Autodesk Inventor part; units mm, degrees
ref_plane "YZ Plane" through (0, 0, 0) normal (1, 0, 0) x (0, 1, 0)
ref_plane "XZ Plane" through (0, 0, 0) normal (0, 1, 0) x (-1, 0, 0)
ref_plane "XY Plane" through (0, 0, 0) normal (0, 0, 1) x (1, 0, 0)
sketch "Sketch1" plane through (0, 0, 0) normal (0, 1, 0) x (-1, 0, 0)
  circle A0 centre (0, 0) radius 3
  line L0 (1.25, 1.75) -> (-1.25, 1.75)
  line L1 (-1.25, 1.75) -> (-1.25, -1.75)
  line L2 (-1.25, -1.75) -> (1.25, -1.75)
  line L3 (1.25, -1.75) -> (1.25, 1.75)
  dimension "d0" = 6
  dimension "d1" = 2.5
  dimension "d2" = 3.5
  dimension "d3" = 1.25
  dimension "d4" = 1.75
extrude "Extrusion1" add sketch "Sketch1" along normal blind 4 contours A0 | L3 L2 L1 L0
extrude "Extrusion2" cut sketch "Sketch1" along normal blind 3 contours L3 L2 L1 L0
fillet "Fillet1" radius 1 1 edges at (3, 4, 0)
properties part number "Power_Button"
For this review, take the finished solid that the model builds, in its own axes (mm). Round coordinates to 2 decimals unless told otherwise and drop trailing zeros. Loops run counter-clockwise (first coordinate to the right, second up) from the corner with the lowest first, then second, coordinate; pieces in that order, holes last. Notation, with made-up numbers: (-1, -0.75) - (15, -0.75) arc R22 cw to (15, 15.25) - close; hole circle Ø4 at (44.5, 32). An arc over 180 degrees is marked (long way). Use one line per item in the form item = value.
1) Mouldability with a two-part tool opening along X and no side actions: class faces 1 (the face through (1.25, 1, 0)), 2 (the face through (0, 4, 0)), 3 (the face through (3, 1, 0)) as pulls with the +X half, pulls with the -X half, needs draft (parallel to the pull), parting line crosses it, or undercut.
Solutions:
face_1 = undercut
face_2 = needs draft
face_3 = parting line crosses it
2) We need section C-C on x = 0. Write out the cut boundary in (y, z), then the cut area to 3 significant figures.
Solutions:
outline = (0, -3) - (3, -3) arc R1 ccw to (4, -2) - (4, 2) arc R1 ccw to (3, 3) - (0, 3) - (0, 1.75) - (3, 1.75) - (3, -1.75) - (0, -1.75) - close
area = 13.1 mm2
3) We need section A-A on y = 1.9. Write out the cut boundary in (x, z).
Solutions:
outline = circle Ø6 at (0, 0); hole (-1.25, -1.75) - (1.25, -1.75) - (1.25, 1.75) - (-1.25, 1.75) - close
4) We need section D-D on y = 3.3. Write out the cut boundary in (x, z), then the cut area to 3 significant figures.
Solutions:
outline = circle Ø5.91 at (0, 0)
area = 27.4 mm2
5) Wall thickness on probe 1 along Z at (x, y) = (0.5, 1.9); probe 2 along X at (y, z) = (1.15, 0.5); probe 3 along Y at (x, z) = (0.5, -1.5): over which ranges is each line inside the solid? List them lowest first.
Solutions:
probe_1 = -2.96 to -1.75, 1.75 to 2.96
probe_2 = -2.96 to -1.25, 1.25 to 2.96
probe_3 = 3 to 4
6) We need section B-B on z = 0. Write out the cut boundary in (x, y), then the cut area to 3 significant figures.
Solutions:
outline = (-3, 0) - (-1.25, 0) - (-1.25, 3) - (1.25, 3) - (1.25, 0) - (3, 0) - (3, 3) arc R1 ccw to (2, 4) - (-2, 4) arc R1 ccw to (-3, 3) - close
area = 16.1 mm2
7) Clearance check with a flat-ended pin moving along its axis: P1, Ø2, axis at x = 0, z = -0.5, coming from the -Y side. State where the tip first meets the part, or that it passes through.
Solutions:
P1 = 3
